```python
from build123d import *

# Parameters (mm, degrees)
F1_DEPTH = 25.4
F2_R     = 12.7
F3_DEPTH = 25.4


with BuildPart() as f1:
    # F0 (on Top) → F1 (new body)
    with BuildSketch(Plane.XY):
        with BuildLine():
            Line((-25.4, 127), (-25.4, 0))
            Line((-25.4, 0), (25.4, 0))
            Line((25.4, 0), (25.4, 127))
            ThreePointArc((25.4, 127), (0, 101.6), (-25.4, 127))
        make_face()
        with BuildLine():
            ThreePointArc((25.4, 127), (0, 152.4), (-25.4, 127))
            Line((-25.4, 127), (25.4, 127))
        make_face()
        with BuildLine():
            Line((25.4, 127), (-25.4, 127))
            ThreePointArc((-25.4, 127), (0, 101.6), (25.4, 127))
        make_face()
    extrude(amount=F1_DEPTH)

    # F2 (on face) → F3 (cut)
    with BuildSketch(Plane.XY.offset(25.4)):
        with Locations((0, 127)):
            Circle(F2_R)
    extrude(amount=-F3_DEPTH, mode=Mode.SUBTRACT)

    # F4: F1 across face


with BuildPart() as f1_1:
    add(f1.part)
    add(f1.part.mirror(Plane(origin=(0, 0, 12.7), x_dir=(1, 0, 0), z_dir=(0, -1, 0))))


solid = f1_1.part
```
Build history of the part. All positions in model axes, mm. Round coordinates to 2 decimals unless told otherwise and drop trailing zeros. Write each loop counter-clockwise with the first axis right and the second up, starting at its lowest first coordinate (ties: lowest second). Pieces come first, ordered by that corner, then holes.
1) Pin check, flat tips, straight feed: pin 1 (1 mm diameter, centred on x = -6.5, z = 21.5, fed in from -Y); pin 2 (3 mm diameter, centred on x = -1.5, y = 1, fed in from -Z). Stop position of each tip, or through.
2) Drill centre lines: probe 1 along Y at (x, z) = (0, 6.5); probe 2 along X at (y, z) = (-127, 8.25); probe 3 along Y at (x, z) = (11.5, 3.5). Where is each one in solid material? Low to high.
3) Mould opens along Z. For faces 1 (the flat face through (0, -2, 0)), 2 (the flat face through (0, -2, 25.4)), 3 (the flat face through (-25.4, -2, 13)) say: +Z half, -Z half, draft (parallel to the pull), parting line (faces both ways), or undercut.
4) Band-saw the part on A-A, the plane x = 0. List the corners of the cut face in (y, z).
5) Band-saw the part on D-D, the plane x = -18.5. List the corners of the cut face in (y, z), and give its area (3 significant figures).
6) Band-saw the part on B-B, the plane z = 21. List the corners of the cut face in (x, y).
7) Band-saw the part on C-C, the plane x = 18. List the corners of the cut face in (y, z).
Ans:
1. pin 1: stops at y = -151.68
1. pin 2: stops at z = 0
2. probe 1: y = -152.4 to -139.7, -114.3 to 114.3, 139.7 to 152.4
2. probe 2: x = -25.4 to -12.7, 12.7 to 25.4
2. probe 3: y = -149.65 to -132.39, -121.61 to 121.61, 132.39 to 149.65
3. face 1: -Z half
3. face 2: +Z half
3. face 3: draft
4. outline: (-152.4, 0) - (-139.7, 0) - (-139.7, 25.4) - (-152.4, 25.4) - close; (-114.3, 0) - (114.3, 0) - (114.3, 25.4) - (-114.3, 25.4) - close; (139.7, 0) - (152.4, 0) - (152.4, 25.4) - (139.7, 25.4) - close
5. outline: (-144.4, 0) - (144.4, 0) - (144.4, 25.4) - (-144.4, 25.4) - close
5. area: 7,340 mm2
6. outline: (-25.4, -127) arc R25.4 ccw to (25.4, -127) - (25.4, 127) arc R25.4 ccw to (-25.4, 127) - close; hole circle Ø25.4 at (0, -127); hole circle Ø25.4 at (0, 127)
7. outline: (-144.92, 0) - (144.92, 0) - (144.92, 25.4) - (-144.92, 25.4) - close
